CAD build for the part. Positions are in the model's coordinates, mm. Round coordinates to 2 decimals unless told otherwise and drop trailing zeros. Order: outer loops, then holes, each group sorted by start corner. A loop starts at its lowest first (then second) coordinate and runs counter-clockwise, first axis right, second up. Notation, with made-up numbers: M -21.75,58.25 L -8.75,58.25 A15 ccw -8.75,77.25 Z; hole C 62.25,80.25 d6. An arc over 180 degrees is marked long. Answer as a JSON object with one key per item and string values.
```python
from build123d import *

# Parameters (mm, degrees)
SKETCH1_W           = 384
SKETCH1_H           = 500
BOSS_EXTRUDE1_DEPTH = 5
SKETCH2_R           = 10
CUT_EXTRUDE1_DEPTH  = 316.379136913


with BuildPart() as part:
    # Sketch1 → Boss-Extrude1 (new, symmetric)
    with BuildSketch(Plane(origin=(0, 0, 0), x_dir=(0, 0, -1), z_dir=(1, 0, 0))):
        Rectangle(SKETCH1_W, SKETCH1_H)
    extrude(amount=BOSS_EXTRUDE1_DEPTH, both=True)

    # Sketch2 → Cut-Extrude1 (cut, through all)
    with BuildSketch(Plane(origin=(5, 0, 0), x_dir=(0, 0, -1), z_dir=(1, 0, 0))):
        with Locations((0, 210)):
            Circle(SKETCH2_R)
    extrude(amount=-CUT_EXTRUDE1_DEPTH, mode=Mode.SUBTRACT)


solid = part.part
```
Item 1: Saw through at B-B on z = 0. List the corners of the cut face in (x, y).
Worked answers:
{"outline": "M -5,-250 L 5,-250 L 5,200 L -5,200 Z; M -5,220 L 5,220 L 5,250 L -5,250 Z"}
Item 2: Drop a flat-ended pin along its axis: pin 1 Ø12 at (y, z) = (210, 0) entering from +X. Give the stop position or say it passes through.
Worked answers:
{"pin 1": "passes through"}
Item 3: Two-plate mould, pull along Z, no slides. Class faces 1 (the cylindrical face through (0.07, 200.24, 2.17)), 2 (the flat face through (-5, 4, 3)), 3 (the flat face through (0, -3, 192)), 4 (the flat face through (0, -3, -192)): released by +Z, released by -Z, zero draft, split by the parting line, or undercut.
Worked answers:
{"face 1": "undercut", "face 2": "zero draft", "face 3": "released by +Z", "face 4": "released by -Z"}
Item 4: Wall check: line 1 along Y through (x, z) = (1.5, 0). Give the ranges that are in metal, low to high. Write a range as [from, to].
Worked answers:
{"line 1": "y = [-250, 200], [220, 250]"}
Item 5: Saw through at A-A on y = 210. List the corners of the cut face in (x, z), and give its area (3 significant figures).
Worked answers:
{"outline": "M -5,-192 L 5,-192 L 5,-10 L -5,-10 Z; M -5,10 L 5,10 L 5,192 L -5,192 Z", "area": "3,640 mm2"}
